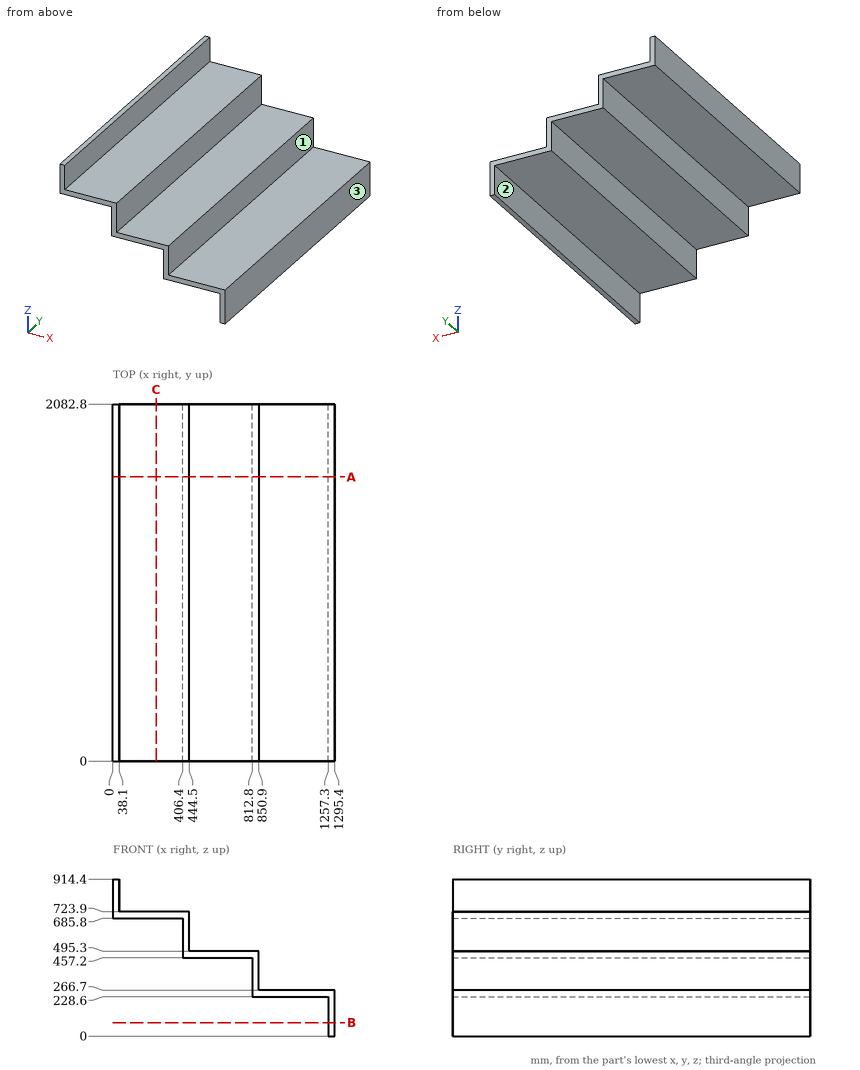
Geometry check sheet. Reference: drawing and pictorial views, mm from the part's lowest x, y, z. A direction names the side the tool comes from. Give positions to 0.01 mm unless a question says otherwise; leave off trailing zeros. Write each loop counter-clockwise with the first axis right and the second up, starting at its lowest first coordinate (ties: lowest second). Pieces come first, ordered by that corner, then holes.
Item 1: Gauge pin test, flat ends, axial feed: pin 1 (6 mm diameter, centred on x = 803, y = 964, fed in from +Z); pin 2 (2 mm diameter, centred on y = 456, z = 765, fed in from +X); pin 3 (1 mm diameter, centred on y = 1488.5, z = 676, fed in from +X). Record the tip position at first contact, or that the pin passes through.
Item 2: Access from +Z, -Z, +X, -X, +Y, -Y to the whole of each face (thin tool, end or side, straight path). Record for the marked faces 1, 2 and 3.
Item 3: Cross-section at C-C (x = 252). Enter the section's corners in (y, z), and give its area (3 significant figures).
Item 4: Cross-section at A-A (y = 1657.5). Enter the section's corners in (x, z).
Item 5: Scan lines: L1, parallel to X at y = 1828, z = 806; L2, parallel to X at y = 897.5, z = 640.5; L3, parallel to Z at x = 587, y = 1136. Record each from-to range of solid material in increasing order.
Item 6: Cross-section at B-B (z = 77.5). Enter the section's corners in (x, y).
Report:
1. pin 1: stops at z = 495.3
1. pin 2: stops at x = 38.1
1. pin 3: stops at x = 444.5
2. face 1: +Z, +X, +Y, -Y
2. face 2: -Z, -X, +Y, -Y
2. face 3: +Z, -Z, +X, +Y, -Y
3. outline: (0, 685.8) - (2082.8, 685.8) - (2082.8, 723.9) - (0, 723.9) - close
3. area: 79,400 mm2
4. outline: (0, 685.8) - (406.4, 685.8) - (406.4, 457.2) - (812.8, 457.2) - (812.8, 228.6) - (1257.3, 228.6) - (1257.3, 0) - (1295.4, 0) - (1295.4, 266.7) - (850.9, 266.7) - (850.9, 495.3) - (444.5, 495.3) - (444.5, 723.9) - (38.1, 723.9) - (38.1, 914.4) - (0, 914.4) - close
5. L1: x = 0 to 38.1
5. L2: x = 406.4 to 444.5
5. L3: z = 457.2 to 495.3
6. outline: (1257.3, 0) - (1295.4, 0) - (1295.4, 2082.8) - (1257.3, 2082.8) - close
